Autodesk Inventor part; units mm, degrees
ref_plane "XZ Plane" through (0, 0, 0) normal (0, 1, 0) x (-1, 0, 0)
ref_plane "XY Plane" through (0, 0, 0) normal (0, 0, 1) x (1, 0, 0)
sketch "Sketch1" plane through (0, 0, 0) normal (0, 0, 1) x (1, 0, 0)
  line L0 (-24.5, 24.5) -> (24.5, 24.5)
  line L1 (24.5, 24.5) -> (24.5, -24.5)
  line L2 (24.5, -24.5) -> (-24.5, -24.5)
  line L3 (-24.5, -24.5) -> (-24.5, 24.5)
  point P0 (0, 0)
  point P1 (-24.5, 0)
  point P2 (0, 24.5)
  dimension "Width" = 49
  dimension "Height" = 49
extrude "Extrusion1" add sketch "Sketch1" along normal blind 20
sketch "Sketch2" plane through (0, 0, 20) normal (0, 0, 1) x (1, 0, 0)
  line L0 (24.5, 24.5) -> (24.5, -24.5)
  line L1 (-24.5, 24.5) -> (24.5, 24.5)
  line L2 (-24.5, -24.5) -> (-24.5, 24.5)
  line L3 (24.5, -24.5) -> (-24.5, -24.5)
  line L4 (19.5, 19.5) -> (19.5, -19.5)
  line L5 (19.5, -19.5) -> (-19.5, -19.5)
  line L6 (-19.5, -19.5) -> (-19.5, 19.5)
  line L7 (-19.5, 19.5) -> (19.5, 19.5)
  point P0 (0, 0)
  dimension "d4" = 5
  dimension "d5" = 39
  dimension "d6" = 39
hole "Hole1" at (-19.5, -19.5, 20) direction (0, 0, -1) diameter 6 end through all
pattern_linear "Rectangular Pattern1" count 2 spacing 39 along (1, 0, 0) count 2 spacing 39 along (0, 1, 0) of "Hole1"
sketch "Sketch3" plane through (0, 0, 0) normal (1, 0, 0) x (0, 1, 0)
  line L0 (-24.5, 20) -> (24.5, 20)
  line L1 (0, 20) -> (0, 28)
  line L2 (0, 28) -> (20.5, 28)
  line L3 (20.5, 28) -> (20.5, 26)
  line L4 (20.5, 26) -> (17.5, 26)
  line L5 (17.5, 26) -> (17.5, 22)
  line L6 (17.5, 22) -> (20.5, 22)
  line L7 (20.5, 22) -> (20.5, 20)
  point P0 (0, 0)
  dimension "d25" = 8
  dimension "d26" = 20.5
  dimension "d27" = 2
  dimension "d28" = 4
  dimension "d29" = 17.5
revolve "Revolution1" add sketch "Sketch3" angle 360 about axis through (0, 0, 20) along (0, 0, 1)
sketch "Sketch4" plane through (-24.5, 24.5, 0) normal (0, 1, 0) x (1, 0, 0)
  line L0 (0, -20) -> (49, -20)
  line L1 (0, 0) -> (0, -20)
  line L2 (24.5, -20) -> (24.5, -14)
  point P0 (24.5, 0)
  dimension "d32" = 6
hole "Hole2" at (0, 0, 28) direction (0, 0, -1) diameter 10 depth 18 counterbore diameter 26 counterbore depth 6
hole "Hole3" at (0, 24.5, 14) direction (0, -1, 0) diameter 4.134 end up to surface
sketch "Sketch6" plane through (24.5, -24.5, 0) normal (1, 0, 0) x (0, 0, -1)
  line L0 (0, 49) -> (0, 0)
  line L1 (0, 49) -> (-20, 49)
  point P0 (0, 24.5)
  point P1 (-10, 24.5)
  point P2 (0, 24.5)
  point P3 (-10, 49)
hole "Hole4" at (24.5, 0, 10) direction (-1, 0, 0) diameter 10 depth 10 tip angle 118
mirror "Mirror1" about plane through (0, 0, 0) normal (1, 0, 0) of "Hole4"
equation "\"Height\" = Width"
equation "\"d16\" = d5"
equation "\"d19\" = d6"
properties part number "TU-001" material "Steel, Mild"
Could you check a few things on this model? Use its own coordinates, in mm. A direction names the side the tool comes from. Round coordinates to 2 decimals unless told otherwise and drop trailing zeros. Loops run counter-clockwise (first coordinate to the right, second up) from the corner with the lowest first, then second, coordinate; pieces in that order, holes last. Notation, with made-up numbers: (72, 37) - (110, 37) arc R11 ccw to (110, 43) - close; hole circle Ø8 at (-24.75, 40). An arc over 180 degrees is marked (long way). Write item = value, one per line.
1) Imagine slicing it at C-C (z = 14). Give the number of separate pieces and of enclosed holes in the cut face, and give its area (3 significant figures).
Computed:
separate_pieces = 1
enclosed_holes = 4
area = 2,000 mm2
2) I'm going to push flat-ended pins straight in: P1, Ø12, axis at x = 2, y = 4, coming from the +Z side; P2, Ø9.5, axis at x = -19.5, y = 19.5, coming from the +Z side; P3, Ø6, axis at x = 0, y = 0, coming from the +Z side; P4, Ø5, axis at x = -19.5, y = -19.5, coming from the -Z side. Where does each tip first touch, or does it pass through?
Computed:
P1 = 22
P2 = 20
P3 = 10
P4 = through
3) If we mould it in two halves opening along Y, with no side actions, what happens to faces 1 (the cylindrical face through (-17.7, 21.9, 9.9)), 2 (the flat face through (-22, 0, 20)), 3 (the flat face through (0, -24.5, 10)), 4 (the cylindrical face through (-10.648, -13.887, 23.972))? For each: pulls with the +Y half, pulls with the -Y half, needs draft (parallel to the pull), parting line crosses it, or undercut.
Computed:
face_1 = undercut
face_2 = needs draft
face_3 = pulls with the -Y half
face_4 = parting line crosses it
4) Imagine slicing it at D-D (x = 6.5). Please give me the cut outline in (y, z).
Computed:
outline = (-24.5, 0) - (24.5, 0) - (24.5, 20) - (19.44, 20) - (19.44, 22) - (16.25, 22) - (16.25, 26) - (19.44, 26) - (19.44, 28) - (11.26, 28) - (11.26, 22) - (-11.26, 22) - (-11.26, 28) - (-19.44, 28) - (-19.44, 26) - (-16.25, 26) - (-16.25, 22) - (-19.44, 22) - (-19.44, 20) - (-24.5, 20) - close
5) On a 3-axis mill with a long thin cutter (end or side, diameter ignored), from which of +Z, -Z, +X, -X, +Y, -Y can I reach the whole of each face in a straight line? I mean faces 5 (the flat face through (-9.2, 15.1, 22)), 6 (the cylindrical face through (19.43, -1.5, 5.23)), 7 (the flat face through (0, -6, 22)), 8 (the cylindrical face through (-19.43, 1.5, 5.23)), 9 (the cylindrical face through (-0.62, 14.39, 15.97)). Say none if no direction works.
Computed:
face_5 = none
face_6 = +X
face_7 = +Z
face_8 = -X
face_9 = +Y
6) Imagine slicing it at A-A (y = 19.5). Please give me the cut outline in (x, z).
Computed:
outline = (-24.5, 0) - (-22.5, 0) - (-22.5, 20) - (-24.5, 20) - close; (-16.5, 0) - (16.5, 0) - (16.5, 20) - (6.32, 20) - (6.32, 22) - (-6.32, 22) - (-6.32, 20) - (-16.5, 20) - close; (-6.32, 26) - (6.32, 26) - (6.32, 28) - (-6.32, 28) - close; (22.5, 0) - (24.5, 0) - (24.5, 20) - (22.5, 20) - close; hole circle Ø4.13 at (0, 14)
7) Imagine slicing it at B-B (x = -19.5). Please give me the cut outline in (y, z).
Computed:
outline = (-24.5, 0) - (-22.5, 0) - (-22.5, 20) - (-24.5, 20) - close; (-16.5, 0) - (16.5, 0) - (16.5, 20) - (6.32, 20) - (6.32, 22) - (-6.32, 22) - (-6.32, 20) - (-16.5, 20) - close; (-6.32, 26) - (6.32, 26) - (6.32, 28) - (-6.32, 28) - close; (22.5, 0) - (24.5, 0) - (24.5, 20) - (22.5, 20) - close; hole circle Ø10 at (0, 10)
8) I need wall thicknesses on line 1 along X through (y, z) = (-19.5, 8); line 2 along Y through (x, z) = (0, 25.35); line 3 along Z through (x, y) = (-17, 0). Which ranges of each line are inside material? Lowest first, please. Write a range as from..to.
Computed:
line_1 = -24.5..-22.5, -16.5..16.5, 22.5..24.5
line_2 = -17.5..-13, 13..17.5
line_3 = 0..5, 15..28
